from build123d import *

# Parameters (mm, degrees)
SKETCH1_W           = 165
SKETCH1_H           = 30
BOSS_EXTRUDE1_DEPTH = 2
FILLET1_R           = 5
SKETCH3_R           = 4
CUT_EXTRUDE1_DEPTH  = 2
SKETCH4_R           = 7.5
CUT_EXTRUDE2_DEPTH  = 10
SKETCH5_R           = 1.5
CUT_EXTRUDE3_DEPTH  = 10
SKETCH6_R           = 1.5
CUT_EXTRUDE4_DEPTH  = 84.876397157


with BuildPart() as part:
    # Sketch1 → Boss-Extrude1 (new body)
    with BuildSketch(Plane(origin=(0, 0, 0), x_dir=(1, 0, 0), z_dir=(0, 1, 0))):
        Rectangle(SKETCH1_W, SKETCH1_H)
    extrude(amount=BOSS_EXTRUDE1_DEPTH)

    # Fillet1
    fillet1_edges = [part.edges().sort_by_distance(p)[0] for p in [
        (82.5, 1, 15),
        (-82.5, 1, 15),
        (-82.5, 1, -15),
        (82.5, 1, -15),
    ]]
    fillet(fillet1_edges, radius=FILLET1_R)

    # Sketch3 → Cut-Extrude1 (cut)
    with BuildSketch(Plane(origin=(0, 2, 0), x_dir=(1, 0, 0), z_dir=(0, 1, 0))):
        with Locations(Location((-67.5, 0, 0), (0, 0, 270))):
            Circle(SKETCH3_R)
    extrude(amount=-CUT_EXTRUDE1_DEPTH, mode=Mode.SUBTRACT)

    # Sketch4 → Cut-Extrude2 (cut)
    with BuildSketch(Plane(origin=(0, 2, 0), x_dir=(1, 0, 0), z_dir=(0, 1, 0))):
        with Locations((82.5, 0)):
            Circle(SKETCH4_R)
    extrude(amount=-CUT_EXTRUDE2_DEPTH, mode=Mode.SUBTRACT)

    # Sketch5 → Cut-Extrude3 (cut)
    with BuildSketch(Plane(origin=(0, 2, 0), x_dir=(1, 0, 0), z_dir=(0, 1, 0))):
        with Locations(Location((-32.5, 10, 0), (0, 0, 270))):
            Circle(SKETCH5_R)
        with Locations(Location((37.5, 10, 0), (0, 0, 270))):
            Circle(SKETCH5_R)
        with Locations(Location((-32.5, -10, 0), (0, 0, 270))):
            Circle(SKETCH5_R)
        with Locations(Location((37.5, -10, 0), (0, 0, 270))):
            Circle(SKETCH5_R)
    extrude(amount=-CUT_EXTRUDE3_DEPTH, mode=Mode.SUBTRACT)

    # Sketch6 → Cut-Extrude4 (cut, through all)
    with BuildSketch(Plane(origin=(0, 2, 0), x_dir=(1, 0, 0), z_dir=(0, 1, 0))):
        with Locations(Location((72.5, 10, 0), (0, 0, 270))):
            Circle(SKETCH6_R)
        with Locations(Location((72.555859106, -10, 0), (0, 0, 270))):
            Circle(SKETCH6_R)
    extrude(amount=-CUT_EXTRUDE4_DEPTH, mode=Mode.SUBTRACT)


solid = part.part
Check sheet for the modelled part. Datum: model origin and axes. Units: mm. Give positions to 0.01 mm unless a question says otherwise; leave off trailing zeros. Write each loop counter-clockwise with the first axis right and the second up, starting at its lowest first coordinate (ties: lowest second). Pieces come first, ordered by that corner, then holes. Notation, with made-up numbers: (25.5, 29) -> (45.5, 29) arc R33 ccw to (45.5, 62) -> close; hole circle Ø6 at (37, 10). An arc over 180 degrees is marked (long way). Write item = value, one per line.
Item 1: Sectioned sample at C-C on y = 0.75. Record the boundary of the cut face in (x, z).
Output:
outline = (-82.5, -10) arc R5 ccw to (-77.5, -15) -> (77.5, -15) arc R5 ccw to (82.5, -10) -> (82.5, -7.5) arc R7.5 cw to (82.5, 7.5) -> (82.5, 10) arc R5 ccw to (77.5, 15) -> (-77.5, 15) arc R5 ccw to (-82.5, 10) -> close; hole circle Ø8 at (-67.5, 0); hole circle Ø3 at (-32.5, -10); hole circle Ø3 at (-32.5, 10); hole circle Ø3 at (37.5, -10); hole circle Ø3 at (37.5, 10); hole circle Ø3 at (72.5, -10); hole circle Ø3 at (72.56, 10)
Item 2: Sectioned sample at A-A on z = 0. Record the boundary of the cut face in (x, y), and give its area (3 significant figures).
Output:
outline = (-82.5, 0) -> (-71.5, 0) -> (-71.5, 2) -> (-82.5, 2) -> close; (-63.5, 0) -> (75, 0) -> (75, 2) -> (-63.5, 2) -> close
area = 299 mm^2
Item 3: Sectioned sample at D-D on z = -6. Record the boundary of the cut face in (x, y).
Output:
outline = (-82.5, 0) -> (78, 0) -> (78, 2) -> (-82.5, 2) -> close
Item 4: Sectioned sample at B-B on x = 37.5. Record the boundary of the cut face in (y, z).
Output:
outline = (0, -15) -> (2, -15) -> (2, -11.5) -> (0, -11.5) -> close; (0, -8.5) -> (2, -8.5) -> (2, 8.5) -> (0, 8.5) -> close; (0, 11.5) -> (2, 11.5) -> (2, 15) -> (0, 15) -> close
Item 5: Release check for a two-part mould opening along X. For faces 1 (the cylindrical face through (-81.07, 1.01, 13.5)), 2 (the cylindrical face through (75, 1, 0)), 3 (the cylindrical face through (36, 1, -10)) record: +X half, -X half, draft (parallel to the pull), parting line (faces both ways), or undercut.
Output:
face_1 = -X half
face_2 = +X half
face_3 = undercut
Item 6: Gauge pin test, flat end, axial feed: pin 1 (2.5 mm diameter, centred on x = 72.5, z = -10, fed in from -Y). Record the tip position at first contact, or that the pin passes through.
Output:
pin_1 = through
Item 7: Scan lines: probe 1 along X at (y, z) = (1, 10); probe 2 along X at (y, z) = (0.5, -10); probe 3 along X at (y, z) = (1.3, 0). Record each from-to range of solid material in increasing order. Write a range as from..to.
Output:
probe_1 = -82.5..-34, -31..36, 39..71.06, 74.06..82.5
probe_2 = -82.5..-34, -31..36, 39..71, 74..82.5
probe_3 = -82.5..-71.5, -63.5..75
